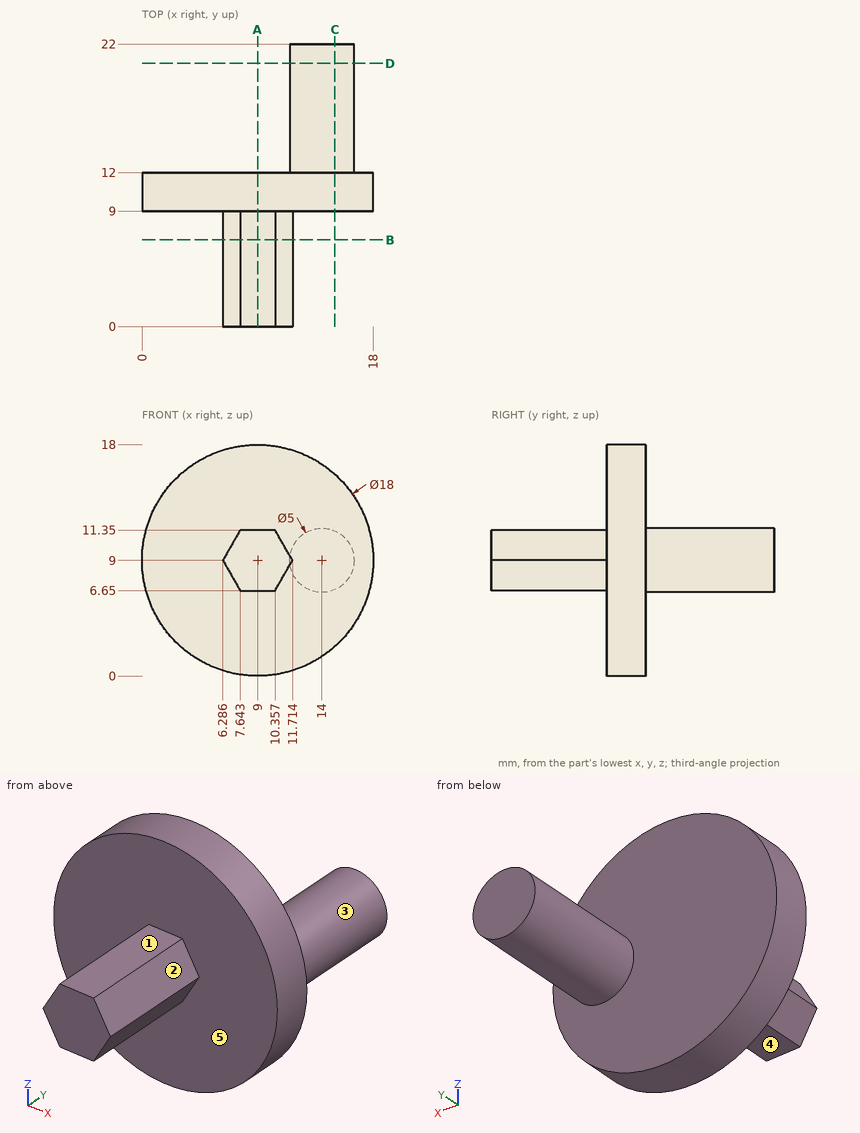
For this review, use the dimensioned drawing (mm, ordinates from the lowest corner) and the shaded views. A direction names the side the tool comes from. Round coordinates to 2 decimals unless told otherwise and drop trailing zeros. Write each loop counter-clockwise with the first axis right and the second up, starting at its lowest first coordinate (ties: lowest second). Pieces come first, ordered by that corner, then holes. Notation, with made-up numbers: (65.5, -30.5) -> (101.5, -30.5) arc R15 cw to (101.5, -19.5) -> close; hole circle Ø1 at (56.25, -2). An arc over 180 degrees is marked (long way). One line per item, written item: value. Start each with the question number.
Q1. Add section C-C (x = 15). Give the boundary of the cut face in (y, z).
Q2. Add section D-D (y = 20.5). Give the boundary of the cut face in (x, z), then the cut area to 3 significant figures.
Q3. To check wall thickness, follow probe 1 along Y at (x, z) = (12.5, 11.25); probe 2 along Z at (x, y) = (7.75, 6); probe 3 along Y at (x, z) = (7.25, 8.5). State the ranges of each line that lie inside material, in increasing order.
Q4. Insertion check: P1, Ø0.8, axis at x = 9, y = 3.5, coming from the -Z side; P2, Ø1, axis at x = 3, y = 13, coming from the +Z side; P3, Ø3, axis at x = 8.5, y = 3.5, coming from the +Z side; P4, Ø2, axis at x = 9, z = 9.5, coming from the +Y side. Each pin has a flat end and moves straight along its axis. Give the tip position at first contact, or say it passes through.
Q5. Add section A-A (x = 9). Give the boundary of the cut face in (y, z).
Q6. Add section B-B (y = 6.75). Give the boundary of the cut face in (x, z).
Q7. Tool access review of the marked faces 1, 2, 3, 4 and 5: name each direction out of +Z, -Z, +X, -X, +Y, -Y from which nothing blocks a thin tool from reaching the whole face with its end or side.
Response:
1. outline: (9, 2.29) -> (12, 2.29) -> (12, 6.71) -> (22, 6.71) -> (22, 11.29) -> (12, 11.29) -> (12, 15.71) -> (9, 15.71) -> close
2. outline: circle Ø5 at (14, 9)
2. area: 19.6 mm^2
3. probe 1: y = 9 to 12
3. probe 2: z = 6.65 to 11.35
3. probe 3: y = 0 to 12
4. P1: stops at z = 6.65
4. P2: passes through
4. P3: stops at z = 11.35
4. P4: stops at y = 12
5. outline: (0, 6.65) -> (9, 6.65) -> (9, 0) -> (12, 0) -> (12, 18) -> (9, 18) -> (9, 11.35) -> (0, 11.35) -> close
6. outline: (6.29, 9) -> (7.64, 6.65) -> (10.36, 6.65) -> (11.71, 9) -> (10.36, 11.35) -> (7.64, 11.35) -> close
7. face 1: +Z, +X, -X, -Y
7. face 2: +Z, +X, -Y
7. face 3: +Y
7. face 4: -Z, +X, -X, -Y
7. face 5: -Y
